The figure shows three views and two pictorial views of one solid part (mm, origin at its lowest corner). Answer the questions. A direction names the side the tool comes from. Coordinates: 2 decimals unless noted, no trailing zeros. Write each loop counter-clockwise with the first axis right and the second up, starting at its lowest first coordinate (ties: lowest second). Pieces come first, ordered by that corner, then holes.
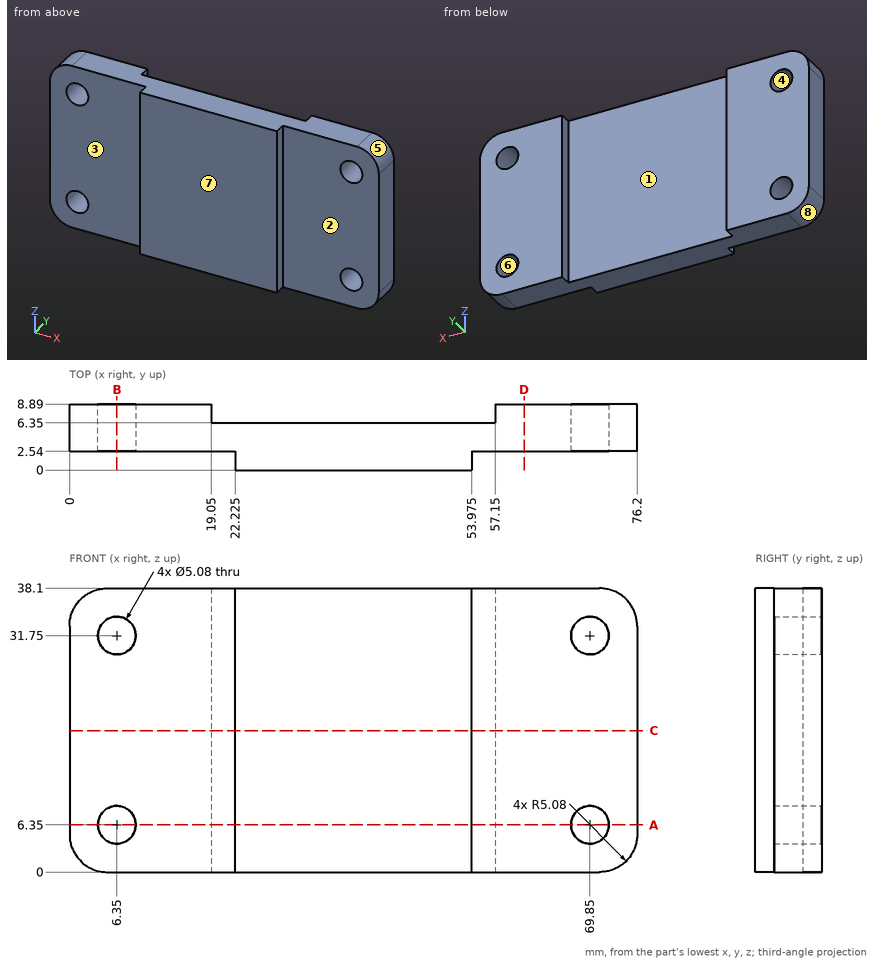
Q1. Given pin 1 (1 mm diameter, centred on x = 68, z = 17.5, fed in from -Y); pin 2 (11.5 mm diameter, centred on x = 35.5, z = 12.5, fed in from +Y); pin 3 (8 mm diameter, centred on x = 6.35, z = 31.75, fed in from +Y); pin 4 (4.5 mm diameter, centred on x = 6.35, z = 6.35, fed in from +Y), each flat-ended and moving along its own axis, determine where each tip first touches the part or whether it passes through.
Answers below:
pin 1: stops at y = 2.54
pin 2: stops at y = 6.35
pin 3: stops at y = 8.89
pin 4: passes through
Q2. Which of the six approach directions +Z, -Z, +X, -X, +Y, -Y give full straight-line access (tool end or side, diameter ignored) to the marked faces 1, 2, 3 and 4?
Answers below:
face 1: +Z, -Z, +Y
face 2: +Z, -Z, +X, -Y
face 3: +Z, -Z, -X, -Y
face 4: +Y, -Y
Q3. The part is cut by section D-D, the plane x = 61. Write down the section's boundary in (y, z), then the cut area to 3 significant figures.
Answers below:
outline: (2.54, 0) - (8.89, 0) - (8.89, 38.1) - (2.54, 38.1) - close
area: 242 mm2
Q4. Determine the mould class of the marked faces 5, 6, 7 and 8 for opening direction X: released by +X, released by -X, zero draft, split by the parting line, or undercut.
Answers below:
face 5: released by +X
face 6: undercut
face 7: zero draft
face 8: released by -X
Q5. The part is cut by section B-B, the plane x = 6.35. Write down the section's boundary in (y, z).
Answers below:
outline: (2.54, 0) - (8.89, 0) - (8.89, 3.81) - (2.54, 3.81) - close; (2.54, 8.89) - (8.89, 8.89) - (8.89, 29.21) - (2.54, 29.21) - close; (2.54, 34.29) - (8.89, 34.29) - (8.89, 38.1) - (2.54, 38.1) - close
Q6. The part is cut by section C-C, the plane z = 19. Write down the section's boundary in (x, y) (3 decimals), then the cut area to 3 significant figures.
Answers below:
outline: (0, 2.54) - (22.225, 2.54) - (22.225, 0) - (53.975, 0) - (53.975, 2.54) - (76.2, 2.54) - (76.2, 8.89) - (57.15, 8.89) - (57.15, 6.35) - (19.05, 6.35) - (19.05, 8.89) - (0, 8.89) - close
area: 468 mm2
Q7. Find the intervals of material crossed by probe 1 along Z at (x, y) = (6.35, 4); probe 2 along X at (y, z) = (8, 28); probe 3 along X at (y, z) = (8.25, 6.5), in increasing order.
Answers below:
probe 1: z = 0 to 3.81, 8.89 to 29.21, 34.29 to 38.1
probe 2: x = 0 to 19.05, 57.15 to 76.2
probe 3: x = 0 to 3.81, 8.89 to 19.05, 57.15 to 67.31, 72.39 to 76.2
Q8. The part is cut by section A-A, the plane z = 6.35. Write down the section's boundary in (x, y) (3 decimals), then the cut area to 3 significant figures.
Answers below:
outline: (0, 2.54) - (3.81, 2.54) - (3.81, 8.89) - (0, 8.89) - close; (8.89, 2.54) - (22.225, 2.54) - (22.225, 0) - (53.975, 0) - (53.975, 2.54) - (67.31, 2.54) - (67.31, 8.89) - (57.15, 8.89) - (57.15, 6.35) - (19.05, 6.35) - (19.05, 8.89) - (8.89, 8.89) - close; (72.39, 2.54) - (76.2, 2.54) - (76.2, 8.89) - (72.39, 8.89) - close
area: 403 mm2
